```python
from build123d import *

# Parameters (mm, degrees)
CROQUIS1_W              = 43
CROQUIS1_H              = 23
SALIENTE_EXTRUIR1_DEPTH = 3
REDONDEO1_R             = 2
CROQUIS2_R              = 10.3
CORTAR_EXTRUIR1_DEPTH   = 2
CROQUIS3_R              = 2.5
CORTAR_EXTRUIR2_DEPTH   = 1


with BuildPart() as part:
    # Croquis1 → Saliente-Extruir1 (new body)
    with BuildSketch(Plane(origin=(0, 0, 0), x_dir=(1, 0, 0), z_dir=(0, 1, 0))):
        Rectangle(CROQUIS1_W, CROQUIS1_H)
    extrude(amount=SALIENTE_EXTRUIR1_DEPTH)

    # Redondeo1
    redondeo1_edges = [part.edges().sort_by_distance(p)[0] for p in [
        (21.5, 1.5, 11.5),
        (-21.5, 1.5, 11.5),
        (-21.5, 1.5, -11.5),
        (21.5, 1.5, -11.5),
    ]]
    fillet(redondeo1_edges, radius=REDONDEO1_R)

    # Croquis2 → Cortar-Extruir1 (cut)
    with BuildSketch(Plane(origin=(0, 3, 0), x_dir=(1, 0, 0), z_dir=(0, 1, 0))):
        with Locations(Location((-10.5, 0, 0), (0, 0, 270))):
            Circle(CROQUIS2_R)
        with Locations(Location((10.5, 0, 0), (0, 0, 90))):
            Circle(CROQUIS2_R)
    extrude(amount=-CORTAR_EXTRUIR1_DEPTH, mode=Mode.SUBTRACT)

    # Croquis3 → Cortar-Extruir2 (cut)
    with BuildSketch(Plane(origin=(0, 1, 0), x_dir=(1, 0, 0), z_dir=(0, 1, 0))):
        with Locations(Location((-10.5, 0, 0), (0, 0, 270))):
            Circle(CROQUIS3_R)
        with Locations(Location((10.5, 0, 0), (0, 0, 270))):
            Circle(CROQUIS3_R)
    extrude(amount=-CORTAR_EXTRUIR2_DEPTH, mode=Mode.SUBTRACT)


solid = part.part
```
Read the model definition and answer for the solid it produces. Units are mm, in the model's axes. A direction names the side the tool comes from. Give positions to 0.01 mm unless a question says otherwise; leave off trailing zeros. Order: outer loops, then holes, each group sorted by start corner. A loop starts at its lowest first (then second) coordinate and runs counter-clockwise, first axis right, second up. Notation, with made-up numbers: (68.5, -6.5) -> (127.5, -6.5) arc R22 cw to (127.5, 19.5) -> close; hole circle Ø4 at (2.5, -20.5). An arc over 180 degrees is marked (long way). Write item = value, one per line.
1. A cutting plane is placed at C-C, the plane y = 2.6. Write down the section's boundary in (x, z), and give its area (3 significant figures).
Numbers:
outline = (-21.5, -9.5) arc R2 ccw to (-19.5, -11.5) -> (19.5, -11.5) arc R2 ccw to (21.5, -9.5) -> (21.5, 9.5) arc R2 ccw to (19.5, 11.5) -> (-19.5, 11.5) arc R2 ccw to (-21.5, 9.5) -> close; hole circle Ø20.6 at (-10.5, 0); hole circle Ø20.6 at (10.5, 0)
area = 319 mm²
2. Given pin 1 (1.5 mm diameter, centred on x = -8, z = -6, fed in from +Y); pin 2 (4 mm diameter, centred on x = 1, z = 2.5, fed in from -Y), each flat-ended and moving along its own axis, determine where each tip first touches the part or whether it passes through.
Numbers:
pin_1 = 1
pin_2 = 0
3. Straight lines are drawn through the part: line 1 along X through (y, z) = (0.35, 0); line 2 along X through (y, z) = (2.2, 0); line 3 along Y through (x, z) = (6.5, -7.75). For each, find the intervals that lie inside material, in ascending order.
Numbers:
line_1 = -21.5 to -13, -8 to 8, 13 to 21.5
line_2 = -21.5 to -20.8, -0.2 to 0.2, 20.8 to 21.5
line_3 = 0 to 1
4. For faces 4 (the face through (20.9, 1.52, 10.93)), 5 (the face through (-20.555, 2.014, -2.233)), determine the directions among +Z, -Z, +X, -X, +Y, -Y from which every point of the face is accessible in a straight line to the end or side of a thin tool.
Numbers:
face_4 = +Z, +X, +Y, -Y
face_5 = +Y
5. The mould has two halves that part along X. Classify faces 1 (the face through (-20.93, 1.52, -10.9)), 2 (the face through (21.5, 1, 0)), 3 (the face through (20.555, 2.014, 2.233)): +X half, -X half, draft (parallel to the pull), parting line (faces both ways), or undercut.
Numbers:
face_1 = -X half
face_2 = +X half
face_3 = undercut
6. A cutting plane is placed at D-D, the plane x = 17. Write down the section's boundary in (y, z), and give its area (3 significant figures).
Numbers:
outline = (0, -11.5) -> (3, -11.5) -> (3, -7.99) -> (1, -7.99) -> (1, 7.99) -> (3, 7.99) -> (3, 11.5) -> (0, 11.5) -> close
area = 37.0 mm²
7. A cutting plane is placed at A-A, the plane z = 0. Write down the section's boundary in (x, y).
Numbers:
outline = (-21.5, 0) -> (-13, 0) -> (-13, 1) -> (-20.8, 1) -> (-20.8, 3) -> (-21.5, 3) -> close; (-8, 0) -> (8, 0) -> (8, 1) -> (0.2, 1) -> (0.2, 3) -> (-0.2, 3) -> (-0.2, 1) -> (-8, 1) -> close; (13, 0) -> (21.5, 0) -> (21.5, 3) -> (20.8, 3) -> (20.8, 1) -> (13, 1) -> close
8. A cutting plane is placed at B-B, the plane x = 10.5. Write down the section's boundary in (y, z), and give its area (3 significant figures).
Numbers:
outline = (0, -11.5) -> (3, -11.5) -> (3, -10.3) -> (1, -10.3) -> (1, -2.5) -> (0, -2.5) -> close; (0, 2.5) -> (1, 2.5) -> (1, 10.3) -> (3, 10.3) -> (3, 11.5) -> (0, 11.5) -> close
area = 22.8 mm²
